Design review of the part built by this model. Coordinates are the model's own, in mm. Coordinates: 2 decimals unless noted, no trailing zeros. Write each loop counter-clockwise with the first axis right and the second up, starting at its lowest first coordinate (ties: lowest second). Pieces come first, ordered by that corner, then holes.
Q1. To check wall thickness, follow probe 1 along Z at (x, y) = (3.25, -2.5); probe 2 along Z at (x, y) = (-2, 0.25); probe 3 along Z at (x, y) = (3.75, 2.75). State the ranges of each line that lie inside material, in increasing order.
Q2. Add section A-A, the plane y = 0. Give the boundary of the cut face in (x, z).
Q3. Clearance check with flat-ended pins moving along their axes: pin 1 Ø1.2 at (y, z) = (-1, 22.5) entering from -X; pin 2 Ø4 at (y, z) = (-4.5, 302) entering from -X; pin 3 Ø6.5 at (x, y) = (-1, 2) entering from -Z. State where each tip first meets the part, or that it passes through.
Q4. Add section B-B, the plane z = 170. Give the boundary of the cut face in (x, y).
from build123d import *

# Parameters (mm, degrees)
SKETCH_2_R               = 3
EXTRUDE_1_DEPTH          = 510
SKETCH_7_R               = 4.5
EXTRUDE_2_DEPTH          = 30
CUT_EXTRUDE_1_DEPTH      = 519.123537392
CUT_EXTRUDE_1_DEPTH_BACK = 519.123537392
EXTRUDE_START            = -30
SKETCH_9_R               = 4.5
EXTRUDE_3_DEPTH          = 30
CUT_EXTRUDE_2_DEPTH      = 30
CUT_EXTRUDE_2_DEPTH_BACK = 30
CUT_EXTRUDE_3_DEPTH      = 30
CUT_EXTRUDE_3_DEPTH_BACK = 30
SKETCH_11_W              = 5.925666616
SKETCH_11_H              = 14.898307071
SKETCH_11_W_2            = 6.139683371
SKETCH_11_W_3            = 15.578698717
SKETCH_11_H_2            = 21.382269556
SKETCH_11_W_4            = 12.448960945


with BuildPart() as part:
    # Sketch 1 → Revolve 4 (revolve)
    with BuildSketch(Plane.XY, mode=Mode.PRIVATE) as revolve_4_sk:
        with BuildLine():
            Line((-7.416198487, 3), (-4, 3))
            ThreePointArc((-4, 3), (-4.472135955, -2.236067977), (0, -5))
            Line((0, -5), (0, -8))
            ThreePointArc((0, -8), (-6.633249581, -4.472135955), (-7.416198487, 3))
        make_face()
    revolve(revolve_4_sk.sketch.rotate(Axis((0, -1000, 0), (0, 1, 0)), 180), axis=Axis((0, -1000, 0), (0, 1, 0)))

    # Sketch 2 → Extrude 1 (add)
    with BuildSketch(Plane.XY):
        with Locations(Location((0, 0, 0), (0, 0, 90))):
            Circle(SKETCH_2_R)
    extrude(amount=EXTRUDE_1_DEPTH)

    # Sketch 4 → Cut-Revolve 1 (revolve, cut)
    with BuildSketch(Plane.XY):
        with BuildLine():
            Line((0, -5), (0, 5))
            ThreePointArc((0, 5), (-5, 0), (0, -5))
        make_face()
    revolve(axis=Axis((0, -1000, 0), (0, 1, 0)), mode=Mode.SUBTRACT)

    # Sketch 6 → Revolve 6 (revolve)
    with BuildSketch(Plane.XY.offset(510), mode=Mode.PRIVATE) as revolve_6_sk:
        with BuildLine():
            Line((-4, 3), (-7.416198487, 3))
            ThreePointArc((-7.416198487, 3), (-6.633249581, -4.472135955), (0, -8))
            Line((0, -8), (0, -5))
            ThreePointArc((0, -5), (-4.472135955, -2.236067978), (-4, 3))
        make_face()
    revolve(revolve_6_sk.sketch.rotate(Axis((0, -1000, 510), (0, 1, 0)), 180), axis=Axis((0, -1000, 510), (0, 1, 0)))

    # Sketch 7 → Extrude 2 (add)
    with BuildSketch(Plane.XY):
        Circle(SKETCH_7_R)
    extrude(amount=EXTRUDE_2_DEPTH)

    # Sketch 8 → Cut-Extrude 1 (cut, two sides: drawn at the far end of the back side and taken through both)
    with BuildSketch(Plane(origin=(0, 0, 0), x_dir=(0, 0, -1), z_dir=(1, 0, 0)).offset(-CUT_EXTRUDE_1_DEPTH_BACK)):
        with BuildLine():
            Line((7.416198487, 3), (-10, 3))
            ThreePointArc((-10, 3), (-11.291313525, 3.41344103), (-12.102370681, 4.5))
            Line((-12.102370681, 4.5), (0, 4.5))
            Line((0, 4.5), (7.416198487, 3))
        make_face()
    extrude(amount=CUT_EXTRUDE_1_DEPTH + CUT_EXTRUDE_1_DEPTH_BACK, mode=Mode.SUBTRACT)

    # Sketch 9 → Extrude 3 (add)
    with BuildSketch(Plane.XY.offset(510).offset(EXTRUDE_START)):
        with Locations(Location((0, 0, 0), (0, 0, 138.189685104))):
            Circle(SKETCH_9_R)
    extrude(amount=EXTRUDE_3_DEPTH)

    # Sketch 10 → Cut-Extrude 2 (cut, two sides: drawn at the far end of the back side and taken through both)
    with BuildSketch(Plane(origin=(0, 0, 0), x_dir=(0, 0, -1), z_dir=(1, 0, 0)).offset(-CUT_EXTRUDE_2_DEPTH_BACK)):
        with BuildLine():
            Line((-522.263931155, 3), (-500, 3))
            ThreePointArc((-500, 3), (-498.712997614, 3.413758441), (-497.908230279, 4.5))
            Line((-497.908230279, 4.5), (-522.188391586, 4.5))
            Line((-522.188391586, 4.5), (-522.263931155, 3))
        make_face()
    extrude(amount=CUT_EXTRUDE_2_DEPTH + CUT_EXTRUDE_2_DEPTH_BACK, mode=Mode.SUBTRACT)

    # Sketch 11 → Cut-Extrude 3 (cut, two sides: drawn at the far end of the back side and taken through both)
    with BuildSketch(Plane(origin=(0, 3, 0), x_dir=(-1, 0, 0), z_dir=(0, 1, 0)).offset(-CUT_EXTRUDE_3_DEPTH_BACK)):
        with Locations((-6.962833308, 482.550846465)):
            Rectangle(SKETCH_11_W, SKETCH_11_H)
        with Locations((7.069841686, 482.550846465)):
            Rectangle(SKETCH_11_W_2, SKETCH_11_H)
        with Locations((-11.789349359, 30.691134778)):
            Rectangle(SKETCH_11_W_3, SKETCH_11_H_2)
        with Locations((10.224480472, 30.691134778)):
            Rectangle(SKETCH_11_W_4, SKETCH_11_H_2)
    extrude(amount=CUT_EXTRUDE_3_DEPTH + CUT_EXTRUDE_3_DEPTH_BACK, mode=Mode.SUBTRACT)


solid = part.part
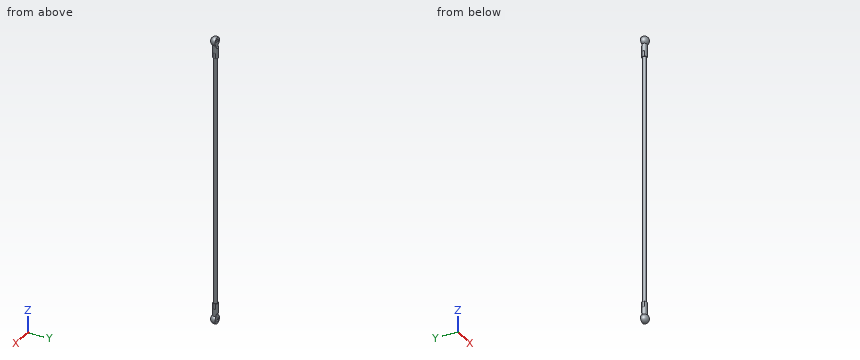
Here are the results:
1. probe 1: z = -6.87 to -2.86, 0 to 30, 480 to 510, 512.86 to 516.87
1. probe 2: z = -7.74 to -4.58, 0 to 510, 514.58 to 517.74
1. probe 3: z = -6.51 to -1.84, 1.84 to 6.51, 503.49 to 508.16, 511.84 to 516.51
2. outline: (-4.5, 6.61) arc R8 ccw (long way) to (4.5, 6.61) - (4.5, 20) - (4, 20) - (4, 30) - (3, 30) - (3, 480) - (4, 480) - (4, 490) - (4.5, 490) - (4.5, 503.39) arc R8 ccw (long way) to (-4.5, 503.39) - (-4.5, 490) - (-4, 490) - (-4, 480) - (-3, 480) - (-3, 30) - (-4, 30) - (-4, 20) - (-4.5, 20) - close; hole (-4.5, 0) - (-4.5, 2.18) arc R5 ccw (long way) to (4.5, 2.18) - (4.5, 0) - close; hole (-4.5, 507.82) - (-4.5, 510) - (4.5, 510) - (4.5, 507.82) arc R5 ccw (long way) to start
3. pin 1: stops at x = -4
3. pin 2: stops at x = -1.66
3. pin 3: stops at z = -8
4. outline: circle Ø6 at (0, 0)
